Design review of the part built by this model. Coordinates are the model's own, in mm. Face numbers are marked on the shaded views. A direction names the side the tool comes from. Give positions to 0.01 mm unless a question says otherwise; leave off trailing zeros. Loops run counter-clockwise (first coordinate to the right, second up) from the corner with the lowest first, then second, coordinate; pieces in that order, holes last. Notation, with made-up numbers: (57.25, -18.5) -> (108.25, -18.5) arc R26 cw to (108.25, -1.5) -> close; hole circle Ø5 at (0.25, 68). An arc over 180 degrees is marked (long way). Answer as CSV lines item,"result".
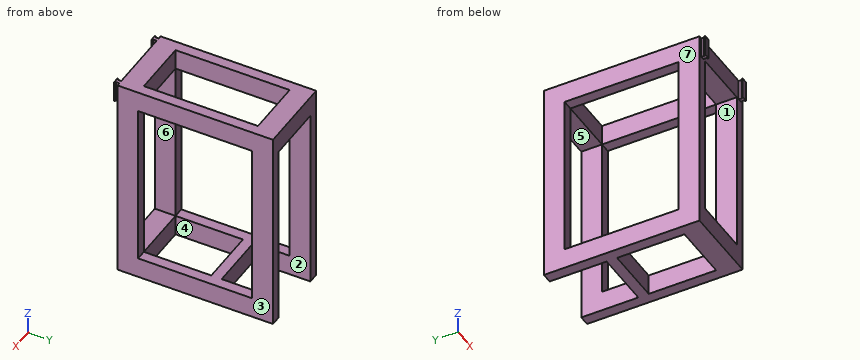
from build123d import *

# Parameters (mm, degrees)
SKETCH3_W           = 190.5
SKETCH3_H           = 508
BOSS_EXTRUDE1_DEPTH = 381
SKETCH4_W           = 406.4
SKETCH4_H           = 279.4
CUT_EXTRUDE1_DEPTH  = 381
SKETCH5_W           = 139.7
SKETCH5_H           = 279.4
CUT_EXTRUDE2_DEPTH  = 924.052
SKETCH6_W           = 139.7
SKETCH6_H           = 406.4
CUT_EXTRUDE3_DEPTH  = 924.052
SKETCH7_W           = 8.89
SKETCH7_H           = 50.8
BOSS_EXTRUDE2_DEPTH = 11.43
SKETCH8_W           = 50.8
SKETCH8_H           = 3.175
BOSS_EXTRUDE3_DEPTH = 3.175
SKETCH9_W           = 50.8
SKETCH9_H           = 3.175
BOSS_EXTRUDE4_DEPTH = 3.175
BOSS_EXTRUDE6_REACH = 488.76
SKETCH11_W          = 50.8
SKETCH11_H          = 25.4
CUT_EXTRUDE4_REACH  = 479.064
SKETCH12_W          = 139.7
SKETCH12_H          = 50.8


with BuildPart() as part:
    # Sketch3 → Boss-Extrude1 (new body)
    with BuildSketch(Plane(origin=(0, 0, 0), x_dir=(1, 0, 0), z_dir=(0, 1, 0))):
        Rectangle(SKETCH3_W, SKETCH3_H)
    extrude(amount=BOSS_EXTRUDE1_DEPTH)

    # Sketch4 → Cut-Extrude1 (cut)
    with BuildSketch(Plane(origin=(95.25, 0, 0), x_dir=(0, 0, -1), z_dir=(1, 0, 0))):
        with Locations((0, 190.5)):
            Rectangle(SKETCH4_W, SKETCH4_H)
    extrude(amount=-CUT_EXTRUDE1_DEPTH, mode=Mode.SUBTRACT)

    # Sketch5 → Cut-Extrude2 (cut)
    with BuildSketch(Plane(origin=(0, 0, -254), x_dir=(-1, 0, 0), z_dir=(0, 0, -1))):
        with Locations((0, 190.5)):
            Rectangle(SKETCH5_W, SKETCH5_H)
    extrude(amount=-CUT_EXTRUDE2_DEPTH, mode=Mode.SUBTRACT)

    # Sketch6 → Cut-Extrude3 (cut)
    with BuildSketch(Plane(origin=(0, 381, 0), x_dir=(1, 0, 0), z_dir=(0, 1, 0))):
        Rectangle(SKETCH6_W, SKETCH6_H)
    extrude(amount=-CUT_EXTRUDE3_DEPTH, mode=Mode.SUBTRACT)

    # Sketch7 → Boss-Extrude2 (add)
    with BuildSketch(Plane.XZ):
        with Locations((-82.55, 228.6)):
            Rectangle(SKETCH7_W, SKETCH7_H)
    boss_extrude2 = extrude(amount=BOSS_EXTRUDE2_DEPTH)

    # Sketch8 → Boss-Extrude3 (add)
    with BuildSketch(Plane(origin=(-78.105, 0, 0), x_dir=(0, 0, -1), z_dir=(1, 0, 0))):
        with Locations((-228.6, -9.8425)):
            Rectangle(SKETCH8_W, SKETCH8_H)
    boss_extrude3 = extrude(amount=BOSS_EXTRUDE3_DEPTH)

    # Sketch9 → Boss-Extrude4 (add)
    with BuildSketch(Plane.ZY.offset(86.995)):
        with Locations((228.6, -9.8425)):
            Rectangle(SKETCH9_W, SKETCH9_H)
    boss_extrude4 = extrude(amount=BOSS_EXTRUDE4_DEPTH)

    # Mirror1: Boss-Extrude2, Boss-Extrude3, Boss-Extrude4 across plane
    add(boss_extrude2.mirror(Plane(origin=(0, 0, 0), x_dir=(0, 0, 1), z_dir=(1, 0, 0))))
    add(boss_extrude3.mirror(Plane(origin=(0, 0, 0), x_dir=(0, 0, 1), z_dir=(1, 0, 0))))
    add(boss_extrude4.mirror(Plane(origin=(0, 0, 0), x_dir=(0, 0, 1), z_dir=(1, 0, 0))))

    # Sketch11 → Boss-Extrude6 (add, up to next)
    with BuildSketch(Plane(origin=(-69.85, 0, 0), x_dir=(0, 0, -1), z_dir=(1, 0, 0)), mode=Mode.PRIVATE) as boss_extrude6_sk1:
        with Locations((228.6, 228.6)):
            Rectangle(SKETCH11_W, SKETCH11_H)
    boss_extrude6_tool1 = extrude(boss_extrude6_sk1.sketch, amount=BOSS_EXTRUDE6_REACH, mode=Mode.PRIVATE) - part.part
    add(boss_extrude6_tool1.solids().sort_by_distance((-69.85, 228.6, -228.6))[0])

    # Sketch12 → Cut-Extrude4 (cut, up to next)
    with BuildSketch(Plane(origin=(0, 381, 0), x_dir=(1, 0, 0), z_dir=(0, 1, 0)), mode=Mode.PRIVATE) as cut_extrude4_sk1:
        with Locations((0, 228.6)):
            Rectangle(SKETCH12_W, SKETCH12_H)
    cut_extrude4_tool1 = extrude(cut_extrude4_sk1.sketch, amount=-CUT_EXTRUDE4_REACH, mode=Mode.PRIVATE) & part.part
    add(cut_extrude4_tool1.solids().sort_by_distance((0, 381, -228.6))[0], mode=Mode.SUBTRACT)


solid = part.part
Q1. For the marked faces 1, 2, 3 and 4, list the 3-axis set-ups (+Z, -Z, +X, -X, +Y, -Y) from which the entire face can be reached by the end or side of a thin tool; tool diameter is ignored.
Filled sheet:
face 1,"+Y, -Y"
face 2,"-Z, +Y"
face 3,"+Z, -Z, +X, +Y, -Y"
face 4,"+Z, -Z"
Q2. We need section C-C, the plane z = -221.5. State the section outline as (x, y) points, and give its area (3 significant figures).
Filled sheet:
outline,"(-95.25, 0) -> (95.25, 0) -> (95.25, 381) -> (69.85, 381) -> (69.85, 241.3) -> (-69.85, 241.3) -> (-69.85, 381) -> (-95.25, 381) -> close; hole (-69.85, 50.8) -> (69.85, 50.8) -> (69.85, 215.9) -> (-69.85, 215.9) -> close"
area,"30,000 mm^2"
Q3. To check wall thickness, follow probe 1 along X at (y, z) = (337, 145.5); probe 2 along Z at (x, y) = (-72, 244); probe 3 along Y at (x, z) = (-16, -211). State the ranges of each line that lie inside material, in increasing order. Write a range as from..to.
Filled sheet:
probe 1,"x = -95.25..-69.85, 69.85..95.25"
probe 2,"z = -254..-203.2, 203.2..254"
probe 3,"y = 0..50.8, 215.9..241.3"
Q4. Clearance check with flat-ended pins moving along their axes: pin 1 Ø3.5 at (y, z) = (-9, 221) entering from -X; pin 2 Ø3.5 at (y, z) = (-10, 233.5) entering from +X; pin 3 Ø4 at (y, z) = (-3.5, 224.5) entering from -X (3 decimals). State where each tip first meets the part, or that it passes through.
Filled sheet:
pin 1,"stops at x = -90.17"
pin 2,"stops at x = 90.17"
pin 3,"stops at x = -86.995"
Q5. The part is to be moulded in two halves that separate along Z. For the marked faces 5, 6 and 7, say which applies: pulls with the +Z half, pulls with the -Z half, needs draft (parallel to the pull), parting line crosses it, or undercut.
Filled sheet:
face 5,"pulls with the -Z half"
face 6,"undercut"
face 7,"needs draft"
Q6. We need section B-B, the plane z = 39.5. State the section outline as (x, y) points.
Filled sheet:
outline,"(-95.25, 0) -> (-69.85, 0) -> (-69.85, 50.8) -> (-95.25, 50.8) -> close; (-95.25, 330.2) -> (-69.85, 330.2) -> (-69.85, 381) -> (-95.25, 381) -> close; (69.85, 0) -> (95.25, 0) -> (95.25, 50.8) -> (69.85, 50.8) -> close; (69.85, 330.2) -> (95.25, 330.2) -> (95.25, 381) -> (69.85, 381) -> close"
Q7. We need section D-D, the plane y = 42. State the section outline as (x, z) points, and give its area (3 significant figures).
Filled sheet:
outline,"(-95.25, -254) -> (95.25, -254) -> (95.25, 254) -> (-95.25, 254) -> close; hole (-69.85, -203.2) -> (69.85, -203.2) -> (69.85, 203.2) -> (-69.85, 203.2) -> close"
area,"40,000 mm^2"
Q8. We need section A-A, the plane y = 309. State the section outline as (x, z) points.
Filled sheet:
outline,"(-95.25, -254) -> (-69.85, -254) -> (-69.85, -203.2) -> (-95.25, -203.2) -> close; (-95.25, 203.2) -> (-69.85, 203.2) -> (-69.85, 254) -> (-95.25, 254) -> close; (69.85, -254) -> (95.25, -254) -> (95.25, -203.2) -> (69.85, -203.2) -> close; (69.85, 203.2) -> (95.25, 203.2) -> (95.25, 254) -> (69.85, 254) -> close"
